Geometry check sheet. Reference: drawing and pictorial views, mm from the part's lowest x, y, z. Round coordinates to 2 decimals unless told otherwise and drop trailing zeros. Write each loop counter-clockwise with the first axis right and the second up, starting at its lowest first coordinate (ties: lowest second). Pieces come first, ordered by that corner, then holes. Notation, with made-up numbers: M -30,31.25 L -23,31.25 A6 cw -23,41.25 Z; hole C 67.25,48 d10. An arc over 180 degrees is marked long. Put each result on its own line as item: value. Start each with the question number.
(1) Mould release check, pull along X, two halves, no side actions. Record for the marked faces 1, 2, 3 and 4: pulls with the +X half, pulls with the -X half, needs draft (parallel to the pull), parting line crosses it, or undercut.
(2) Section check C-C on y = 37. Record the cut outline in (x, z) (1 decimal).
(3) Gauge pin test, flat ends, axial feed: pin 1 (5 mm diameter, centred on x = 32, z = 23, fed in from +Y); pin 2 (2 mm diameter, centred on x = 76, y = 36, fed in from -Z); pin 3 (2 mm diameter, centred on y = 15, z = 42.5, fed in from +X) (1 decimal); pin 4 (5 mm diameter, centred on x = 14.5, z = 43.5, fed in from -Y). Record the tip position at first contact, or that the pin passes through.
(4) Section check B-B on z = 28.5. Record the cut outline in (x, y), then the cut area to 3 significant figures.
(5) Section check A-A on x = 52. Record the cut outline in (y, z) (1 decimal), then the cut area to 3 significant figures.
(6) Material ranges on probe 1 along X at (y, z) = (31.5, 31) (1 decimal); probe 2 along Y at (x, z) = (64, 4); probe 3 along X at (y, z) = (24, 30.5), recorded low to high.
(7) Section check D-D on x = 71.5. Record the cut outline in (y, z), then the cut area to 3 significant figures.
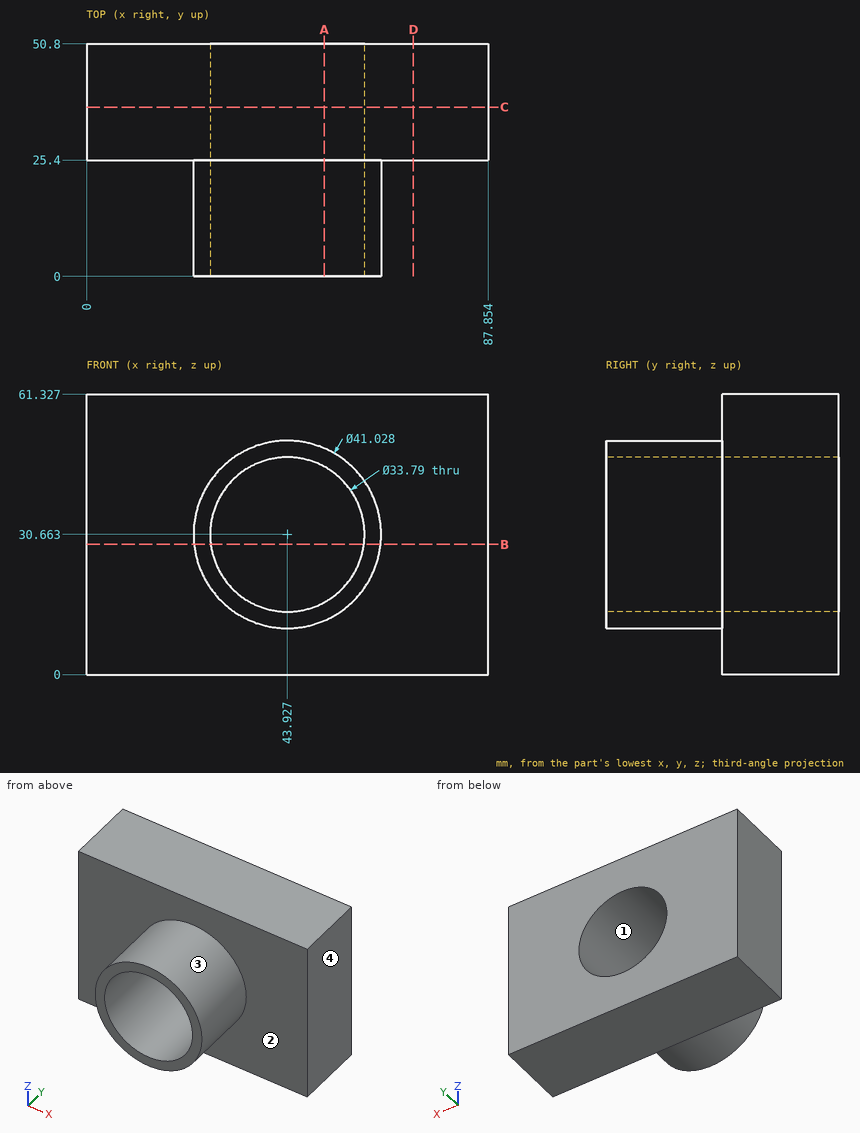
Answers follow:
1. face 1: undercut
1. face 2: needs draft
1. face 3: parting line crosses it
1. face 4: pulls with the +X half
2. outline: M 0,0 L 87.9,0 L 87.9,61.3 L 0,61.3 Z; hole C 43.9,30.7 d33.8
3. pin 1: passes through
3. pin 2: stops at z = 0
3. pin 3: stops at x = 61.3
3. pin 4: stops at y = 25.4
4. outline: M 0,25.4 L 23.53,25.4 L 23.53,0 L 27.17,0 L 27.17,50.8 L 0,50.8 Z; M 60.68,0 L 64.33,0 L 64.33,25.4 L 87.85,25.4 L 87.85,50.8 L 60.68,50.8 Z
4. area: 1,570 mm^2
5. outline: M 0,11.8 L 25.4,11.8 L 25.4,0 L 50.8,0 L 50.8,15.8 L 0,15.8 Z; M 0,45.5 L 50.8,45.5 L 50.8,61.3 L 25.4,61.3 L 25.4,49.5 L 0,49.5 Z
5. area: 1,010 mm^2
6. probe 1: x = 0 to 27, 60.8 to 87.9
6. probe 2: y = 25.4 to 50.8
6. probe 3: x = 23.41 to 27.03, 60.82 to 64.44
7. outline: M 25.4,0 L 50.8,0 L 50.8,61.33 L 25.4,61.33 Z
7. area: 1,560 mm^2
